Build history of the part. All positions in model axes, mm. A direction names the side the tool comes from. Give positions to 0.01 mm unless a question says otherwise; leave off trailing zeros. Order: outer loops, then holes, each group sorted by start corner. A loop starts at its lowest first (then second) coordinate and runs counter-clockwise, first axis right, second up. Notation, with made-up numbers: (-30, 50) - (-22, 50) arc R17 ccw to (-22, 78) - close; hole circle Ø9 at (1, 17). An arc over 180 degrees is marked (long way). Use a Markdown table: item, result.
from build123d import *

# Parameters (mm, degrees)
SALIENTE_EXTRUIR1_DEPTH      = 6.35
TALADRO_DE_MARGEN_PARA_M41_D = 4.5
REDONDEO1_R                  = 5


with BuildPart() as part:
    # Croquis1 → Saliente-Extruir1 (new body)
    with BuildSketch(Plane(origin=(0, 0, 0), x_dir=(0, 0, -1), z_dir=(1, 0, 0))):
        Polygon((-22.5, 85), (-22.5, -35), (22.5, -35), (22.5, 85), (37.5, 85), (37.5, 35), (37.5, -35), (37.5, -85), (22.5, -85), (22.5, -55), (-22.5, -55), (-22.5, -85), (-37.5, -85), (-37.5, -35), (-37.5, 35), (-37.5, 85), align=None)
    extrude(amount=SALIENTE_EXTRUIR1_DEPTH)

    # Taladro de margen para M41 (through all)
    with Locations(Plane.ZY):
        with Locations((30, 68), (30, 80), (-30, 68), (-30, 80), (30, -80), (30, -68), (-30, -80), (-30, -68)):
            Hole(TALADRO_DE_MARGEN_PARA_M41_D / 2)

    # Redondeo1
    redondeo1_edges = [part.edges().sort_by_distance(p)[0] for p in [
        (3.175, 85, 22.5),
        (3.175, 85, -22.5),
        (3.175, 85, -37.5),
        (3.175, -85, -37.5),
        (3.175, -85, -22.5),
        (3.175, -85, 22.5),
        (3.175, -85, 37.5),
        (3.175, 85, 37.5),
    ]]
    fillet(redondeo1_edges, radius=REDONDEO1_R)


solid = part.part
1) Wall check: line 1 (Y direction, x = 5.25, z = -30); line 2 (Z direction, x = 2, y = -3); line 3 (Z direction, x = 2.75, y = -67.5). Give the ranges that are in metal, low to high. Write a range as from..to.
Computed:
| item | result |
|---|---|
| line 1 | y = -85..-82.25, -77.75..-70.25, -65.75..65.75, 70.25..77.75, 82.25..85 |
| line 2 | z = -37.5..-22.5, 22.5..37.5 |
| line 3 | z = -37.5..-32.19, -27.81..-22.5, 22.5..27.81, 32.19..37.5 |
2) Pin check, flat tips, straight feed: P1, Ø7, axis at y = 68, z = 30, coming from the -X side; P2, Ø3, axis at x = 1, z = -7.5, coming from the -Y side; P3, Ø3, axis at x = 3, z = 5, coming from the +Y side. Stop position of each tip, or through.
Computed:
| item | result |
|---|---|
| P1 | stops at x = 0 |
| P2 | stops at y = -55 |
| P3 | stops at y = -35 |
3) Slice it at A-A (y = 14). Write the cut outline in (x, z), and give its area (4 significant figures).
Computed:
| item | result |
|---|---|
| outline | (0, -37.5) - (6.35, -37.5) - (6.35, -22.5) - (0, -22.5) - close; (0, 22.5) - (6.35, 22.5) - (6.35, 37.5) - (0, 37.5) - close |
| area | 190.5 mm² |
4) Slice it at B-B (x = 3). State how many separate pieces and enclosed holes the cut face has, and give its area (3 significant figures).
Computed:
| item | result |
|---|---|
| separate pieces | 1 |
| enclosed holes | 8 |
| area | 5,830 mm² |
5) Two-plate mould, pull along Z, no slides. Class faces 1 (the flat face through (3, 23, 22.5)), 2 (the cylindrical face through (3.22, 83.57, -36)), 3 (the flat face through (6.35, 1, 24)): +Z half, -Z half, draft (parallel to the pull), parting line (faces both ways), or undercut.
Computed:
| item | result |
|---|---|
| face 1 | undercut |
| face 2 | -Z half |
| face 3 | draft |
6) Tool access for faces 4 (the cylindrical face through (3.219, -70.196, -29.512)), 5 (the flat face through (3, 22, -22.5)), 6 (the flat face through (3, -67, 22.5)): list every direction of +Z, -Z, +X, -X, +Y, -Y with a clear straight run to the whole face (end or side of a thin tool).
Computed:
| item | result |
|---|---|
| face 4 | +X, -X |
| face 5 | +X, -X, +Y |
| face 6 | +X, -X, -Y |
7) Slice it at C-C (y = 68). Write the cut outline in (x, z), and give its area (3 significant figures).
Computed:
| item | result |
|---|---|
| outline | (0, -37.5) - (6.35, -37.5) - (6.35, -32.25) - (0, -32.25) - close; (0, -27.75) - (6.35, -27.75) - (6.35, -22.5) - (0, -22.5) - close; (0, 22.5) - (6.35, 22.5) - (6.35, 27.75) - (0, 27.75) - close; (0, 32.25) - (6.35, 32.25) - (6.35, 37.5) - (0, 37.5) - close |
| area | 133 mm² |
8) Slice it at D-D (z = 7). Write the cut outline in (x, y), and give its area (3 significant figures).
Computed:
| item | result |
|---|---|
| outline | (0, -55) - (6.35, -55) - (6.35, -35) - (0, -35) - close |
| area | 127 mm² |
